Autodesk Inventor part; units mm, degrees
ref_plane "YZ Plane" through (0, 0, 0) normal (1, 0, 0) x (0, 1, 0)
ref_plane "XZ Plane" through (0, 0, 0) normal (0, 1, 0) x (-1, 0, 0)
ref_plane "XY Plane" through (0, 0, 0) normal (0, 0, 1) x (1, 0, 0)
sketch "Skizze1" plane through (0, 0, 0) normal (0, 0, 1) x (1, 0, 0)
  circle A0 centre (0, 0) radius 15.5
  dimension "d0" = 31
extrude "Extrusion1" add sketch "Skizze1" along normal blind 12
sketch "Skizze2" plane through (0, 0, 12) normal (0, 0, 1) x (1, 0, 0)
  line L0 (-2.5, -2.5) -> (2.5, -2.5)
  line L1 (2.5, -2.5) -> (2.5, 2.5)
  line L2 (2.5, 2.5) -> (-2.5, 2.5)
  line L3 (-2.5, 2.5) -> (-2.5, -2.5)
  line L4 (-2.5, -2.5) -> (2.5, 2.5) construction
  line L5 (2.5, -2.5) -> (-2.5, 2.5) construction
  point P0 (0, 0)
  dimension "d3" = 5
extrude "Extrusion2" cut sketch "Skizze2" against normal blind 5
sketch "Skizze3" plane through (0, 0, 12) normal (0, 0, 1) x (1, 0, 0)
  circle A0 centre (0, 0) radius 11.25
  line L0 (-7.955, -7.955) -> (7.955, -7.955)
  line L1 (7.955, -7.955) -> (7.955, 7.955)
  line L2 (7.955, 7.955) -> (-7.955, 7.955)
  line L3 (-7.955, 7.955) -> (-7.955, -7.955)
  line L4 (-7.955, -7.955) -> (7.955, 7.955) construction
  line L5 (7.955, -7.955) -> (-7.955, 7.955) construction
  dimension "d6" = 22.5
hole "Bohrung1" at (-7.955, -7.955, 12) at (7.955, -7.955, 12) at (7.955, 7.955, 12) at (-7.955, 7.955, 12) direction (0, 0, -1) diameter 3 end through all counterbore diameter 6 counterbore depth 6
properties part number "rotBaseMagnetMountQube"
Verification items for the finished model (mm, model axes). A direction names the side the tool comes from. Coordinates: 2 decimals unless noted, no trailing zeros. Loops run counter-clockwise (first coordinate to the right, second up) from the corner with the lowest first, then second, coordinate; pieces in that order, holes last. Notation, with made-up numbers: M -11,61 L 4,61 A19 ccw 4,70 Z; hole C -16,78.5 d9. An arc over 180 degrees is marked long. One line per item, written item: value.
1. Section check D-D on y = 0. Record the cut outline in (x, z), plus the area to 3 significant figures.
Answers follow:
outline: M -15.5,0 L 15.5,0 L 15.5,12 L 2.5,12 L 2.5,7 L -2.5,7 L -2.5,12 L -15.5,12 Z
area: 347 mm^2
2. Material ranges on line 1 along Y through (x, z) = (8, 7); line 2 along X through (y, z) = (-8, 2.75); line 3 along X through (y, z) = (-8.5, 1.25), recorded low to high. Write a range as from..to.
Answers follow:
line 1: -13.28..-10.95, -4.96..4.96, 10.95..13.28
line 2: -13.28..-9.45, -6.46..6.46, 9.45..13.28
line 3: -12.96..-9.35, -6.56..6.56, 9.35..12.96
3. Section check C-C on z = 1.5. Record the cut outline in (x, y) (3 decimals).
Answers follow:
outline: C 0,0 d31; hole C -7.955,-7.955 d3; hole C -7.955,7.955 d3; hole C 7.955,-7.955 d3; hole C 7.955,7.955 d3
4. Section check A-A on x = -7.5. Record the cut outline in (y, z), plus the area to 3 significant figures.
Answers follow:
outline: M -13.56,0 L -9.38,0 L -9.38,6 L -10.92,6 L -10.92,12 L -13.56,12 Z; M -6.53,0 L 6.53,0 L 6.53,6 L 4.99,6 L 4.99,12 L -4.99,12 L -4.99,6 L -6.53,6 Z; M 9.38,0 L 13.56,0 L 13.56,12 L 10.92,12 L 10.92,6 L 9.38,6 Z
area: 220 mm^2
5. Section check B-B on y = 8.5. Record the cut outline in (x, z).
Answers follow:
outline: M -12.96,0 L -9.35,0 L -9.35,6 L -10.91,6 L -10.91,12 L -12.96,12 Z; M -6.56,0 L 6.56,0 L 6.56,6 L 5,6 L 5,12 L -5,12 L -5,6 L -6.56,6 Z; M 9.35,0 L 12.96,0 L 12.96,12 L 10.91,12 L 10.91,6 L 9.35,6 Z
6. Gauge pin test, flat ends, axial feed: P1, Ø1.5, axis at y = -1, z = 6, coming from the +X side; P2, Ø1.8, axis at x = 7.5, y = -6.5, coming from the +Z side; P3, Ø1.5, axis at x = -4.5, z = 1.5, coming from the +Y side. Record the tip position at first contact, or that the pin passes through.
Answers follow:
P1: x = 15.5
P2: z = 6
P3: y = 15.04
7. Set-up check for faces 4 (the cylindrical face through (-7.38, -9.34, 2.96)), 5 (the flat face through (2.5, 0, 10)): record each of +Z, -Z, +X, -X, +Y, -Y from which the full face is reachable in a straight line by a thin tool's end or side.
Answers follow:
face 4: +Z, -Z
face 5: +Z
8. Mould release check, pull along X, two halves, no side actions. Record for faces 1 (the flat face through (-6.7, -9.2, 6)), 2 (the flat face through (0, 0, 0)), 3 (the cylindrical face through (-2.018, -15.368, 5.916)): pulls with the +X half, pulls with the -X half, needs draft (parallel to the pull), parting line crosses it, or undercut.
Answers follow:
face 1: undercut
face 2: needs draft
face 3: parting line crosses it
